Geometry: see drawing. Coordinates: mm, zero at the bounding-box minimum. A direction names the side the tool comes from. Round coordinates to 2 decimals unless told otherwise and drop trailing zeros. Order: outer loops, then holes, each group sorted by start corner. A loop starts at its lowest first (then second) coordinate and runs counter-clockwise, first axis right, second up.
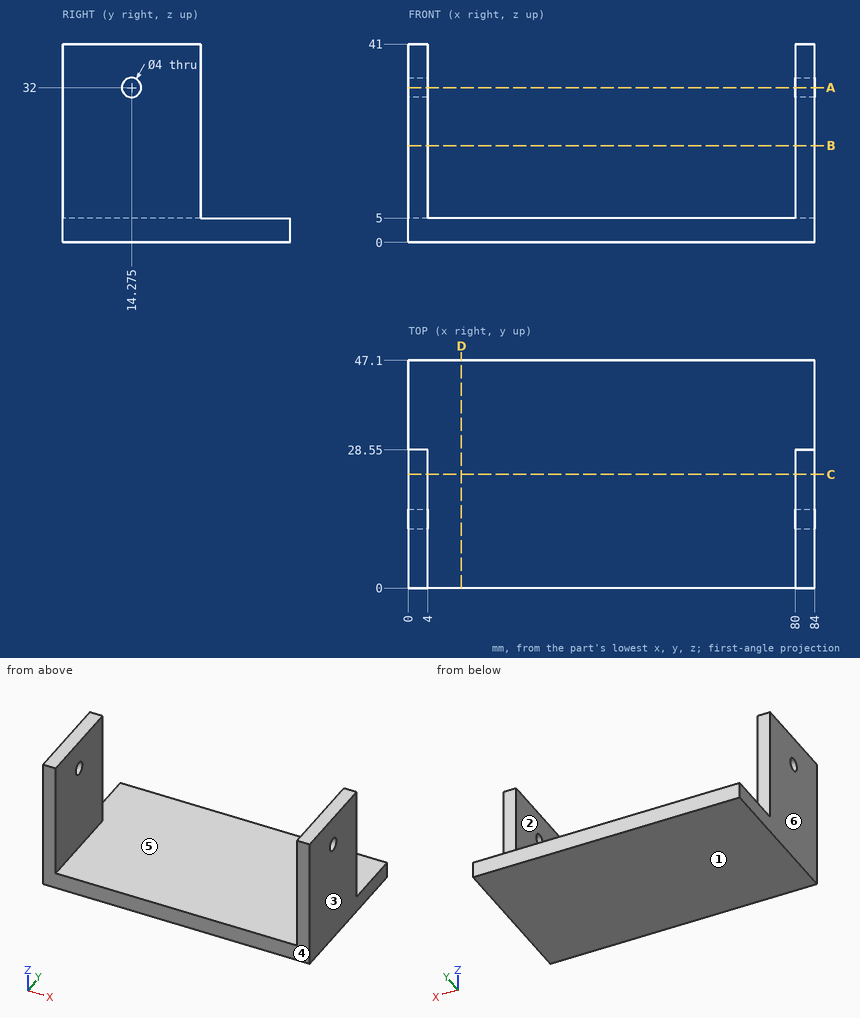
1. Line query: line 1 along X through (y, z) = (21, 25); line 2 along Y through (x, z) = (81.05, 32) (3 decimals); line 3 along Z through (x, y) = (56.5, 38.5). Output: solid intervals per line, ascending.
2. Section D-D on x = 11. Return loops of the section in (y, z).
3. Section A-A on z = 32. Return loops of the section in (x, y) (3 decimals).
4. Pull-direction query (X, two-part tool) for the marked faces 3, 4, 5 and 6; classes: released by +X, released by -X, zero draft, split by the parting line, or undercut.
5. Section C-C on y = 23.5. Return loops of the section in (x, z).
6. Access query for the marked faces 1 and 2. Directions: +Z, -Z, +X, -X, +Y, -Y. A direction counts if a zero-diameter tool reaches every point of the face in a straight line with its end or side. Return the directions, or none.
7. First-contact query: pin 1 (4.5 mm diameter, centred on x = 82.5, z = 22, fed in from +Y); pin 2 (8 mm diameter, centred on x = 18.5, y = 35, fed in from +Z). Flat tips, straight axial feed; report the tip coordinate or a pass-through.
8. Section B-B on z = 20. Return loops of the section in (x, y), plus the area to 3 significant figures.
Result:
1. line 1: x = 0 to 4, 80 to 84
1. line 2: y = 0 to 12.275, 16.275 to 28.55
1. line 3: z = 0 to 5
2. outline: (0, 0) - (47.1, 0) - (47.1, 5) - (0, 5) - close
3. outline: (0, 0) - (4, 0) - (4, 12.275) - (0, 12.275) - close; (0, 16.275) - (4, 16.275) - (4, 28.55) - (0, 28.55) - close; (80, 0) - (84, 0) - (84, 12.275) - (80, 12.275) - close; (80, 16.275) - (84, 16.275) - (84, 28.55) - (80, 28.55) - close
4. face 3: released by +X
4. face 4: zero draft
4. face 5: undercut
4. face 6: released by -X
5. outline: (0, 0) - (84, 0) - (84, 41) - (80, 41) - (80, 5) - (4, 5) - (4, 41) - (0, 41) - close
6. face 1: -Z, +X, -X, +Y, -Y
6. face 2: +Z, +Y, -Y
7. pin 1: stops at y = 28.55
7. pin 2: stops at z = 5
8. outline: (0, 0) - (4, 0) - (4, 28.55) - (0, 28.55) - close; (80, 0) - (84, 0) - (84, 28.55) - (80, 28.55) - close
8. area: 228 mm2
